from build123d import *

# Parameters (mm, degrees)
EXTRUDE_1_DEPTH                   = 10
HOLE_WIZARD_4_1_4_1_1_D           = 4.1
HOLE_WIZARD_4_1_4_1_1_CSINK_D     = 4.15
HOLE_WIZARD_4_1_4_1_1_CSINK_ANGLE = 90
SKETCH_4_R                        = 3.75
EXTRUDE_2_DEPTH                   = 10
FILLET_1_R                        = 0.5
CHAMFER_1_SIZE                    = 1


with BuildPart() as part:
    # 草图1 → 凸台-拉伸1 (new, symmetric)
    with BuildSketch(Plane(origin=(0, 0, 0), x_dir=(1, 0, 0), z_dir=(0, 1, 0))):
        Polygon((0, 0), (-21.721638066, 0), (-21.721638066, -5), (-1.721638066, -5), (12.681907696, -16.253283275), (15.760215072, -12.313229507), align=None)
    extrude(amount=EXTRUDE_1_DEPTH, both=True)

    # Ø4.1 (4.1) 直径孔1 (through all)
    with Locations(Plane(origin=(-19.221638066, 7.5, 5), x_dir=(1, 0, 0), z_dir=(0, 0, 1))):
        with Locations((0, 0), (15, 0), (15, -15), (0, -15)):
            CounterSinkHole(HOLE_WIZARD_4_1_4_1_1_D / 2, HOLE_WIZARD_4_1_4_1_1_CSINK_D / 2, counter_sink_angle=HOLE_WIZARD_4_1_4_1_1_CSINK_ANGLE)

    # 草图4 → 凸台-拉伸2 (add)
    with BuildSketch(Plane(origin=(0, 0, 0), x_dir=(-0.7880107536067258, 0, -0.6156614753256534), z_dir=(0.6156614753256534, 0, -0.7880107536067258))):
        with Locations(Location((-10, 0, 0), (0, 0, 180))):
            Circle(SKETCH_4_R)
    extrude(amount=EXTRUDE_2_DEPTH)

    # 圆角1
    fillet_1_edges = [part.edges().sort_by_distance(p)[0] for p in [
        (11.081681963, 0, -4.032223315),
    ]]
    fillet(fillet_1_edges, radius=FILLET_1_R)

    # 倒角1
    chamfer_1_edges = [part.edges().sort_by_distance(p)[0] for p in [
        (14.221061384, 10, 14.283256391),
        (14.221061384, -10, 14.283256391),
    ]]
    chamfer(chamfer_1_edges, length=CHAMFER_1_SIZE)


solid = part.part
Geometry check sheet. Reference: the model listing, model coordinates, mm. A direction names the side the tool comes from. Round coordinates to 2 decimals unless told otherwise and drop trailing zeros. Order: outer loops, then holes, each group sorted by start corner. A loop starts at its lowest first (then second) coordinate and runs counter-clockwise, first axis right, second up. Notation, with made-up numbers: M 3,5 L 62,5 A24 cw 62,31 Z; hole C 14,20.25 d3. An arc over 180 degrees is marked long. Answer in a Markdown table with one row per item. Add a question column.
Item 1: Sectioned sample at A-A, the plane y = -7.5. Enter the section's corners in (x, z) (3 decimals), plus the area to 3 significant figures.
Item 2: Sectioned sample at D-D, the plane z = 14. Enter the section's corners in (x, y), plus the area to 3 significant figures.
Item 3: Sectioned sample at B-B, the plane y = 5. Enter the section's corners in (x, z), plus the area to 3 significant figures.
Item 4: Draft check along X on faces 1 (the face through (-3.78, -9.5, 2.45)), 2 (the face through (-17.174, 7.59, 2.453)), 3 (the face through (5.38, 0.14, 10.55)), 4 (the face through (-3, -10, 4)). Enter one of: released by +X, released by -X, zero draft, split by the parting line, or undercut.
Item 5: Depth check by flat-ended pin: pin 1 Ø4.5 at (x, y) = (-19.22, 7.5) entering from +Z; pin 2 Ø5 at (x, y) = (-0.5, -7.5) entering from -Z; pin 3 Ø3 at (y, z) = (4, 12.5) entering from +X. Enter the tip coordinate at first touch or a pass-through.
Item 6: Material ranges on L1, parallel to X at y = -7.5, z = 3.15; L2, parallel to X at y = 8.5, z = 2.25; L3, parallel to Z at x = -17.5, y = 1.5, recorded low to high. Write a range as [from, to].
Item 7: Sectioned sample at C-C, the plane x = -9. Enter the section's corners in (y, z), plus the area to 3 significant figures.
Item 8: Set-up check for faces 5 (the face through (-11, 0, 0)), 6 (the face through (-12, 0, 5)), 7 (the face through (7.99, 4.58, 6.24)): record each of +Z, -Z, +X, -X, +Y, -Y from which the full face is reachable in a straight line by a thin tool's end or side.
Filled in:
| question | item | result |
|---|---|---|
| 1 | outline | M -21.722,0 L -21.272,0 L -21.272,4.975 L -21.297,5 L -21.722,5 Z; M -17.172,0 L -6.272,0 L -6.272,4.975 L -6.297,5 L -17.147,5 L -17.172,4.975 Z; M -2.172,0 L 0,0 L 15.76,12.313 L 12.682,16.253 L -1.722,5 L -2.147,5 L -2.172,4.975 Z |
| 1 | area | 159 mm² |
| 2 | outline | M 9.8,-10 L 13.17,-10 L 14.44,-9 L 14.44,9 L 13.17,10 L 9.8,10 Z |
| 2 | area | 91.6 mm² |
| 3 | outline | M -21.72,0 L 0,0 L 15.76,12.31 L 12.68,16.25 L -1.72,5 L -21.72,5 Z |
| 3 | area | 200 mm² |
| 4 | face 1 | undercut |
| 4 | face 2 | undercut |
| 4 | face 3 | released by -X |
| 4 | face 4 | zero draft |
| 5 | pin 1 | stops at z = 5 |
| 5 | pin 2 | stops at z = 0 |
| 5 | pin 3 | stops at x = 15.76 |
| 6 | L1 | x = [-21.72, -21.27], [-17.17, -6.27], [-2.17, 4.03] |
| 6 | L2 | x = [-21.72, -21.01], [-17.43, -6.01], [-2.43, 2.88] |
| 6 | L3 | z = [0, 5] |
| 7 | outline | M -10,0 L 10,0 L 10,5 L -10,5 Z |
| 7 | area | 100 mm² |
| 8 | face 5 | -Z, -X, +Y, -Y |
| 8 | face 6 | +Z, -X, +Y, -Y |
| 8 | face 7 | none |
